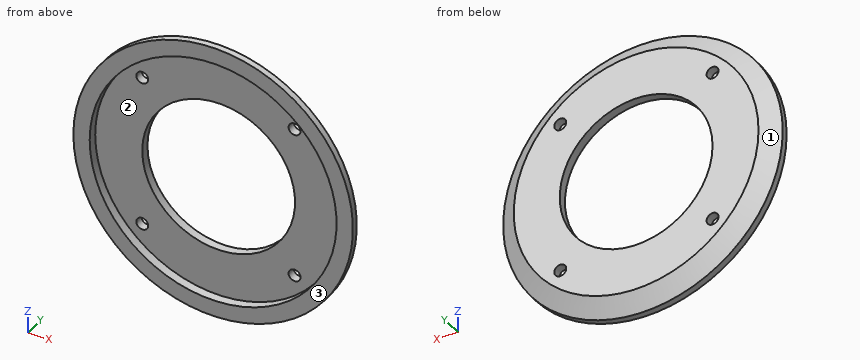
```python
from build123d import *

# Parameters (mm, degrees)
SKETCH_2_R          = 5.5
CUT_EXTRUDE_1_DEPTH = 10


with BuildPart() as part:
    # 草图1 → 旋转1 (revolve)
    with BuildSketch(Plane.XY):
        Polygon((-84.972745292, -8.788732394), (-127.222745292, -8.788732394), (-143.222745292, -19.288732394), (-143.222745292, -25.288732394), (-128.222745292, -25.288732394), (-128.222745292, -16.788732394), (-84.972745292, -16.788732394), align=None)
    revolve(axis=Axis((-14.722745292, 34.411267606, 0), (0, -1, 0)))

    # 草图2 → 切除-拉伸1 (cut)
    with BuildSketch(Plane.XZ.offset(16.788732394)):
        with Locations(Location((-84.972745292, 70, 0), (0, 0, 270))):
            Circle(SKETCH_2_R)
        with Locations(Location((55.027254708, 70, 0), (0, 0, 270))):
            Circle(SKETCH_2_R)
        with Locations(Location((55.027254708, -70, 0), (0, 0, 270))):
            Circle(SKETCH_2_R)
        with Locations(Location((-84.972745292, -70, 0), (0, 0, 270))):
            Circle(SKETCH_2_R)
    extrude(amount=-CUT_EXTRUDE_1_DEPTH, mode=Mode.SUBTRACT)


solid = part.part
```
Build history of the part. All positions in model axes, mm. Face numbers are marked on the shaded views. Round coordinates to 2 decimals unless told otherwise and drop trailing zeros. Loops run counter-clockwise (first coordinate to the right, second up) from the corner with the lowest first, then second, coordinate; pieces in that order, holes last.
Item 1: Two-plate mould, pull along Z, no slides. Class the marked faces 1, 2 and 3: released by +Z, released by -Z, zero draft, split by the parting line, or undercut.
Item 2: Pin check, flat tips, straight feed: P1, Ø8, axis at x = 49.5, y = -23, coming from the -Z side; P2, Ø12.5, axis at x = -84.97, z = -70, coming from the +Y side; P3, Ø17.5, axis at x = 55.03, z = -70, coming from the -Y side; P4, Ø3, axis at x = -76.5, y = -12, coming from the +Z side. Stop position of each tip, or through.
Item 3: Saw through at A-A (z = 0). List the corners of the cut face in (x, y).
Item 4: Saw through at B-B (y = -11.5). List the corners of the cut face in (x, z), then the cut area to 3 significant figures.
Item 5: Drill centre lines: line 1 along Z through (x, y) = (57.5, -10.25); line 2 along Y through (x, z) = (-17, 87.5); line 3 along X through (y, z) = (-17.5, 88). Where is each one in solid material? Low to high.
Worked answers:
1. face 1: split by the parting line
1. face 2: undercut
1. face 3: zero draft
2. P1: stops at z = -113.51
2. P2: stops at y = -8.79
2. P3: stops at y = -16.79
2. P4: stops at z = 102.65
3. outline: (-143.22, -25.29) - (-128.22, -25.29) - (-128.22, -16.79) - (-84.97, -16.79) - (-84.97, -8.79) - (-127.22, -8.79) - (-143.22, -19.29) - close; (55.53, -16.79) - (98.78, -16.79) - (98.78, -25.29) - (113.78, -25.29) - (113.78, -19.29) - (97.78, -8.79) - (55.53, -8.79) - close
4. outline: circle Ø233.26 at (-14.72, 0); hole circle Ø11 at (-84.97, -70); hole circle Ø11 at (-84.97, 70); hole circle Ø140.5 at (-14.72, 0); hole circle Ø11 at (55.03, -70); hole circle Ø11 at (55.03, 70)
4. area: 26,900 mm2
5. line 1: z = -89.14 to -74.91, -65.09 to 65.09, 74.91 to 89.14
5. line 2: y = -16.79 to -8.79
5. line 3: x = -104.58 to -86.4, 56.96 to 75.14
